For this review, use the dimensioned drawing (mm, ordinates from the lowest corner) and the shaded views. Coordinates: 2 decimals unless noted, no trailing zeros. Order: outer loops, then holes, each group sorted by start corner. A loop starts at its lowest first (then second) coordinate and runs counter-clockwise, first axis right, second up. Notation, with made-up numbers: M 58,17.5 L 78,17.5 A19 cw 78,41.5 Z; hole C 56.25,-37.5 d10. An arc over 180 degrees is marked long. Answer in a Markdown table with one row per item.
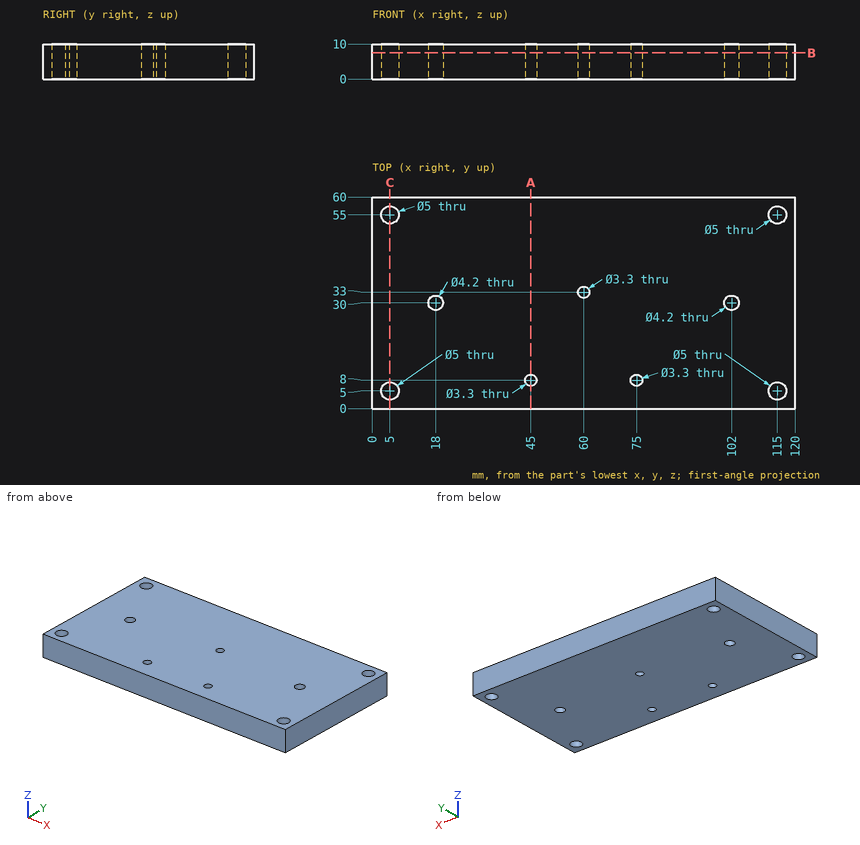
(1) Add section B-B, the plane z = 7.5. Give the number of separate pieces and of enclosed holes in the cut face, and give its area (3 significant figures).
Return value:
| item | result |
|---|---|
| separate pieces | 1 |
| enclosed holes | 9 |
| area | 7,070 mm2 |
(2) Add section C-C, the plane x = 5. Give the boundary of the cut face in (y, z).
Return value:
| item | result |
|---|---|
| outline | M 0,0 L 2.5,0 L 2.5,10 L 0,10 Z; M 7.5,0 L 52.5,0 L 52.5,10 L 7.5,10 Z; M 57.5,0 L 60,0 L 60,10 L 57.5,10 Z |
(3) For line 1 along Y through (x, z) = (115, 4.75); line 2 along X through (y, z) = (7, 7); line 3 along X through (y, z) = (9, 1), list the stretches that pass through material, from the lowest coordinate up. Write a range as from..to.
Return value:
| item | result |
|---|---|
| line 1 | y = 0..2.5, 7.5..52.5, 57.5..60 |
| line 2 | x = 0..3.5, 6.5..43.69, 46.31..73.69, 76.31..113.5, 116.5..120 |
| line 3 | x = 0..43.69, 46.31..73.69, 76.31..120 |
(4) Add section A-A, the plane x = 45. Give the boundary of the cut face in (y, z), and give its area (3 significant figures).
Return value:
| item | result |
|---|---|
| outline | M 0,0 L 6.35,0 L 6.35,10 L 0,10 Z; M 9.65,0 L 60,0 L 60,10 L 9.65,10 Z |
| area | 567 mm2 |
(5) Insertion check: pin 1 Ø5.5 at (x, y) = (102, 30) entering from +Z; pin 2 Ø2.5 at (x, y) = (60, 33) entering from +Z. Each pin has a flat end and moves straight along its axis. Give the tip position at first contact, or say it passes through.
Return value:
| item | result |
|---|---|
| pin 1 | stops at z = 10 |
| pin 2 | passes through |
